For this review, take the finished solid that the model builds, in its own axes (mm). Round coordinates to 2 decimals unless told otherwise and drop trailing zeros. Order: outer loops, then holes, each group sorted by start corner. A loop starts at its lowest first (then second) coordinate and runs counter-clockwise, first axis right, second up. Notation, with made-up numbers: (31, -16) -> (52, -16) arc R18 cw to (52, 18) -> close; hole circle Ø1 at (29, -35). An arc over 180 degrees is marked (long way). Answer in a Markdown table with one row per item.
```python
from build123d import *

# Parameters (mm, degrees)
SKETCH1_W           = 450.85
SKETCH1_H           = 88.9
BOSS_EXTRUDE1_DEPTH = 25.4
CUT_EXTRUDE1_DEPTH  = 51.8


with BuildPart() as part:
    # Sketch1 → Boss-Extrude1 (new body, symmetric)
    with BuildSketch(Plane(origin=(0, 0, 0), x_dir=(1, 0, 0), z_dir=(0, 1, 0))):
        Rectangle(SKETCH1_W, SKETCH1_H)
    extrude(amount=BOSS_EXTRUDE1_DEPTH, both=True)

    # Sketch2 → Cut-Extrude1 (cut, through all)
    with BuildSketch(Plane(origin=(0, 25.4, 0), x_dir=(1, 0, 0), z_dir=(0, 1, 0))):
        Polygon((-225.425, 44.45), (-225.425, -19.05), (-161.925, 44.45), align=None)
        Polygon((225.425, -19.05), (161.925, 44.45), (225.425, 44.45), align=None)
    extrude(amount=-CUT_EXTRUDE1_DEPTH, mode=Mode.SUBTRACT)


solid = part.part
```
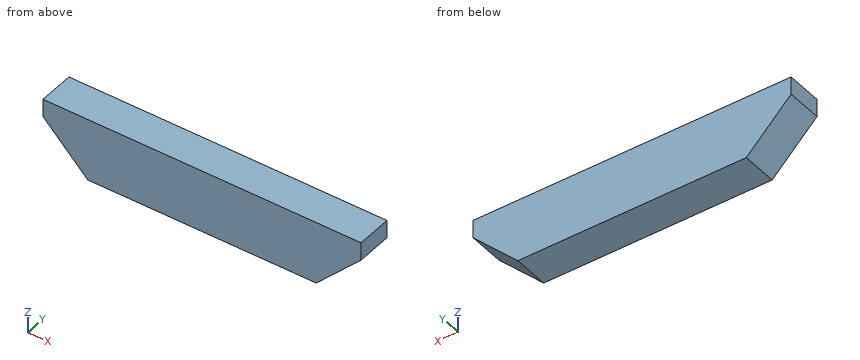
Q1. Take a section at C-C, the plane x = -183.5. Write out the cut boundary in (y, z) (3 decimals), then the cut area to 3 significant figures.
Answer key:
| item | result |
|---|---|
| outline | (-25.4, -22.875) -> (25.4, -22.875) -> (25.4, 44.45) -> (-25.4, 44.45) -> close |
| area | 3,420 mm^2 |
Q2. Clearance check with flat-ended pins moving along their axes: pin 1 Ø3 at (y, z) = (-8.5, -33) entering from +X (3 decimals); pin 2 Ø1.5 at (y, z) = (3.5, -27) entering from +X (3 decimals). State where each tip first meets the part, or that it passes through.
Answer key:
| item | result |
|---|---|
| pin 1 | stops at x = 174.875 |
| pin 2 | stops at x = 180.125 |
Q3. Take a section at A-A, the plane y = -20. Write out the cut boundary in (x, z) (3 decimals), then the cut area to 3 significant figures.
Answer key:
| item | result |
|---|---|
| outline | (-225.425, 19.05) -> (-161.925, -44.45) -> (161.925, -44.45) -> (225.425, 19.05) -> (225.425, 44.45) -> (-225.425, 44.45) -> close |
| area | 36,000 mm^2 |
Q4. To check wall thickness, follow probe 1 along X at (y, z) = (-7, -16.5) (3 decimals); probe 2 along Z at (x, y) = (205.5, -19) (3 decimals); probe 3 along X at (y, z) = (11.5, -32) (3 decimals). State the ranges of each line that lie inside material, in increasing order.
Answer key:
| item | result |
|---|---|
| probe 1 | x = -189.875 to 189.875 |
| probe 2 | z = -0.875 to 44.45 |
| probe 3 | x = -174.375 to 174.375 |
Q5. Take a section at B-B, the plane z = -36. Write out the cut boundary in (x, y) (3 decimals), then the cut area to 3 significant figures.
Answer key:
| item | result |
|---|---|
| outline | (-170.375, -25.4) -> (170.375, -25.4) -> (170.375, 25.4) -> (-170.375, 25.4) -> close |
| area | 17,300 mm^2 |
